For this review, use the dimensioned drawing (mm, ordinates from the lowest corner) and the shaded views. A direction names the side the tool comes from. Give positions to 0.01 mm unless a question says otherwise; leave off trailing zeros. Write each loop counter-clockwise with the first axis right and the second up, starting at its lowest first coordinate (ties: lowest second). Pieces come first, ordered by that corner, then holes.
1) We need section D-D on x = 141.5. Give the boundary of the cut face in (y, z).
2) Wall thickness on line 1 along Z through (x, y) = (76.2, 40); line 2 along X through (y, z) = (30, 93.5); line 3 along Z through (x, y) = (54, 38.5): over which ranges is each line inside the solid? List them lowest first.
3) We need section B-B on y = 12. Give the boundary of the cut face in (x, z).
4) We need section A-A on z = 91. Give the boundary of the cut face in (x, y).
5) For P1, Ø1, axis at x = 94.5, y = 22.5, coming from the +Z side; P2, Ø4, axis at y = 15.5, z = 127.5, coming from the +X side; P3, Ø10, axis at x = 121.5, y = 23, coming from the +Z side, all flat-tipped, find the tip position at first contact; note any pin that passes through.
6) Draft analysis for pull direction X (two halves, no side actions). For the marked faces 1, 2, 3 and 4, state which applies: pulls with the +X half, pulls with the -X half, needs draft (parallel to the pull), parting line crosses it, or undercut.
7) Machinability: for the marked faces 5 and 6, which of the approach directions +Z, -Z, +X, -X, +Y, -Y give a long, thin tool a straight path to every point of the face, cutting with its end or side? Answer none if there is none.
8) We need section C-C on z = 61. Give the boundary of the cut face in (x, y).
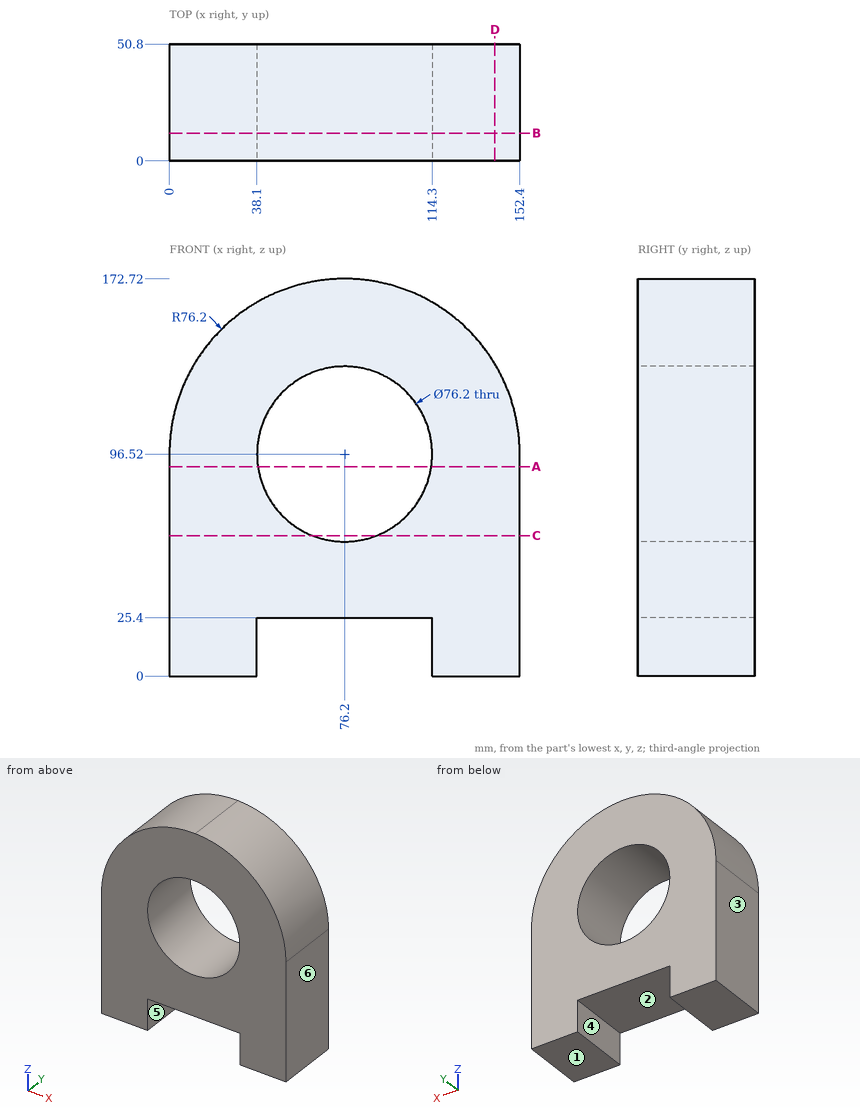
Results list:
1. outline: (0, 0) - (50.8, 0) - (50.8, 135.79) - (0, 135.79) - close
2. line 1: z = 25.4 to 58.42, 134.62 to 172.72
2. line 2: x = 0 to 38.22, 114.18 to 152.4
2. line 3: z = 25.4 to 65.56, 127.48 to 169.41
3. outline: (0, 0) - (38.1, 0) - (38.1, 25.4) - (114.3, 25.4) - (114.3, 0) - (152.4, 0) - (152.4, 96.52) arc R76.2 ccw to (0, 96.52) - close; hole circle Ø76.2 at (76.2, 96.52)
4. outline: (0, 0) - (38.5, 0) - (38.5, 50.8) - (0, 50.8) - close; (113.9, 0) - (152.4, 0) - (152.4, 50.8) - (113.9, 50.8) - close
5. P1: stops at z = 170.61
5. P2: stops at x = 146.67
5. P3: stops at z = 161.19
6. face 1: needs draft
6. face 2: undercut
6. face 3: pulls with the -X half
6. face 4: undercut
7. face 5: -Z, +Y, -Y
7. face 6: +Z, -Z, +X, +Y, -Y
8. outline: (0, 0) - (62.42, 0) - (62.42, 50.8) - (0, 50.8) - close; (89.98, 0) - (152.4, 0) - (152.4, 50.8) - (89.98, 50.8) - close
